Source: CAD feature listing. Evaluate the final solid. Frame: model axes, mm. Give positions to 0.01 mm unless a question says otherwise; leave off trailing zeros. Loops run counter-clockwise (first coordinate to the right, second up) from the corner with the lowest first, then second, coordinate; pieces in that order, holes last.
Autodesk Inventor part; units mm, degrees
ref_plane "YZ Plane" through (0, 0, 0) normal (1, 0, 0) x (0, 1, 0)
ref_plane "XZ Plane" through (0, 0, 0) normal (0, 1, 0) x (-1, 0, 0)
ref_plane "XY Plane" through (0, 0, 0) normal (0, 0, 1) x (1, 0, 0)
sketch "Sketch1" plane through (0, 0, 0) normal (1, 0, 0) x (0, 1, 0)
  circle A0 centre (0, 0) radius 4
  circle A1 centre (0, 0) radius 5
  dimension "d0" = 8
  dimension "d1" = 10
extrude "Extrusion1" add sketch "Sketch1" along normal blind 2
chamfer "Chamfer1" distance 0.25 angle 45 4 edges at (2, -5, 0) (0, -5, 0) (0, -4, 0) (2, -4, 0)
thread "Thread1"
properties part number "Component 30(Intake Pipe Ring)"
(1) Section A-A, the plane y = 0. Return the cut outline in (x, z), then the cut area to 3 significant figures.
A:
outline: (0, -4.75) - (0.25, -5) - (1.75, -5) - (2, -4.75) - (2, -4.25) - (1.75, -4) - (0.25, -4) - (0, -4.25) - close; (0, 4.25) - (0.25, 4) - (1.75, 4) - (2, 4.25) - (2, 4.75) - (1.75, 5) - (0.25, 5) - (0, 4.75) - close
area: 3.75 mm2
(2) Section C-C, the plane x = 0.85. Return the cut outline in (y, z).
A:
outline: circle Ø10 at (0, 0); hole circle Ø8 at (0, 0)
(3) Ray query, line 1 along Z through (x, y) = (1.05, 0); line 2 along Y through (x, z) = (1.4, -2.25); line 3 along Y through (x, z) = (0.3, -3.25). Return the intervals inside material, ascending.
A:
line 1: z = -5 to -4, 4 to 5
line 2: y = -4.47 to -3.31, 3.31 to 4.47
line 3: y = -3.8 to -2.33, 2.33 to 3.8
(4) Mould query, pull axis Z, two halves, no side actions, for faces 1 (the flat face through (2, -4, -2)), 2 (the cylindrical face through (0.99, -1.08, 4.88)), 3 (the cylindrical face through (0.99, -0.867, 3.905)). Classes: pulls with the +Z half, pulls with the -Z half, needs draft (parallel to the pull), parting line crosses it, or undercut.
A:
face 1: needs draft
face 2: parting line crosses it
face 3: undercut
